```python
from build123d import *

# Parameters (mm, degrees)
BOSS_EXTRU_2_DEPTH        = 6.35
ESQUISSE29_R              = 5
BOSS_EXTRU_3_DEPTH        = 6.35
SYM_TRIE2_COPY_1_SKETCH_R = 5
SYM_TRIE2_COPY_1_DEPTH    = 6.35
ESQUISSE30_R              = 1.5
ENL_V_MAT_EXTRU_1_DEPTH   = 41.953581056


with BuildPart() as part:
    # Esquisse28 → Boss.-Extru.2 (new body)
    with BuildSketch(Plane.XY):
        Polygon((-18.97, -25.475382387), (-25.475382387, -18.97), (-25.475382387, 18.97), (-18.97, 25.475382387), (18.97, 25.475382387), (25.475382387, 18.97), (25.475382387, -18.97), (18.97, -25.475382387), align=None)
        Polygon((-16.97, -20.645541049), (-20.645541049, -16.97), (-20.645541049, 16.97), (-16.97, 20.645541049), (16.97, 20.645541049), (20.645541049, 16.97), (20.645541049, -16.97), (16.97, -20.645541049), align=None, mode=Mode.SUBTRACT)
    extrude(amount=BOSS_EXTRU_2_DEPTH)

    # Esquisse29 → Boss.-Extru.3 (add)
    with BuildSketch(Plane.XY):
        with Locations((23.60833184, 23.60833184)):
            Circle(ESQUISSE29_R)
    boss_extru_3 = extrude(amount=BOSS_EXTRU_3_DEPTH)

    # Symétrie1: Boss.-Extru.3 across plane
    add(boss_extru_3.mirror(Plane(origin=(0, 0, 0), x_dir=(0, 0, 1), z_dir=(1, 0, 0))))

    # Symétrie2: Boss.-Extru.3 across plane
    add(boss_extru_3.mirror(Plane.ZX))

    # Symétrie2 copy 1 sketch → Symétrie2 copy 1 (add)
    with BuildSketch(Plane(origin=(0, 0, 0), x_dir=(-1, 0, 0), z_dir=(0, 0, 1))):
        with Locations((23.60833184, 23.60833184)):
            Circle(SYM_TRIE2_COPY_1_SKETCH_R)
    extrude(amount=SYM_TRIE2_COPY_1_DEPTH)

    # Esquisse30 → Enlèv. mat.-Extru.1 (cut, through all)
    with BuildSketch(Plane.XY.offset(6.35)):
        with Locations((-23.60833184, 23.60833184)):
            Circle(ESQUISSE30_R)
        with Locations((23.60833184, 23.60833184)):
            Circle(ESQUISSE30_R)
        with Locations((23.60833184, -23.60833184)):
            Circle(ESQUISSE30_R)
        with Locations((-23.60833184, -23.60833184)):
            Circle(ESQUISSE30_R)
    extrude(amount=-ENL_V_MAT_EXTRU_1_DEPTH, mode=Mode.SUBTRACT)


solid = part.part
```
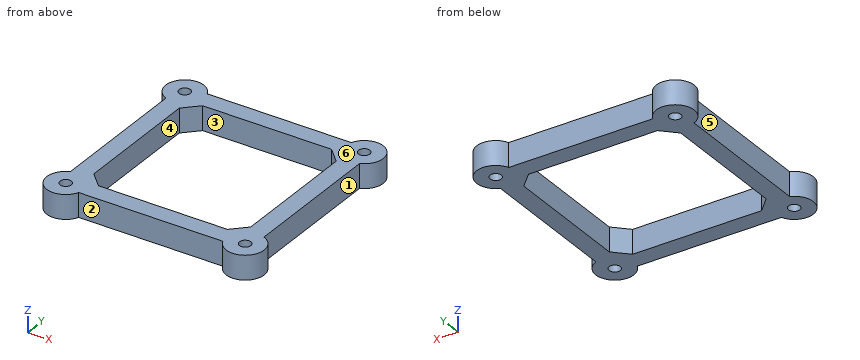
Model file for the job. Use its own axes, mm. Face numbers are marked on the shaded views. A direction names the side the tool comes from. Give positions to 0.01 mm unless a question says otherwise; leave off trailing zeros. Order: outer loops, then holes, each group sorted by start corner. A loop starts at its lowest first (then second) coordinate and runs counter-clockwise, first axis right, second up.
1) Wall check: probe 1 along X at (y, z) = (23.5, 4.75); probe 2 along X at (y, z) = (-15, 2.5). Give the ranges that are in metal, low to high.
2) Saw through at A-A, the plane y = 11. Write the cut outline in (x, z).
3) Pin check, flat tips, straight feed: pin 1 (3 mm diameter, centred on y = -8.5, z = 3.5, fed in from -X); pin 2 (1.8 mm diameter, centred on x = 23.61, y = 23.61, fed in from +Z); pin 3 (2 mm diameter, centred on x = -17.5, z = 2.5, fed in from +Y); pin 4 (5 mm diameter, centred on x = -23.61, y = 23.61, fed in from +Z). Stop position of each tip, or through.
4) Mould opens along X. For the marked faces 4, 5 and 6 say: +X half, -X half, draft (parallel to the pull), parting line (faces both ways), or undercut.
5) Saw through at C-C, the plane z = 2.75. Write the cut outline in (x, y), then the cut area to 3 significant figures.
6) 3-axis set-ups, long thin cutter, end or side, ignore diameter. For the marked faces 1, 2 and 3: which of +Z, -Z, +X, -X, +Y, -Y reach the whole face in a straight line?
Computed:
1. probe 1: x = -28.61 to -25.1, -22.11 to 22.11, 25.1 to 28.61
1. probe 2: x = -25.48 to -20.65, 20.65 to 25.48
2. outline: (-25.48, 0) - (-20.65, 0) - (-20.65, 6.35) - (-25.48, 6.35) - close; (20.65, 0) - (25.48, 0) - (25.48, 6.35) - (20.65, 6.35) - close
3. pin 1: stops at x = -25.48
3. pin 2: passes through
3. pin 3: stops at y = 25.48
3. pin 4: stops at z = 6.35
4. face 4: undercut
4. face 5: -X half
4. face 6: draft
5. outline: (-25.48, -18.97) arc R5 ccw (long way) to (-18.97, -25.48) - (18.97, -25.48) arc R5 ccw (long way) to (25.48, -18.97) - (25.48, 18.97) arc R5 ccw (long way) to (18.97, 25.48) - (-18.97, 25.48) arc R5 ccw (long way) to (-25.48, 18.97) - close; hole circle Ø3 at (-23.61, -23.61); hole circle Ø3 at (-23.61, 23.61); hole (-20.65, -16.97) - (-16.97, -20.65) - (16.97, -20.65) - (20.65, -16.97) - (20.65, 16.97) - (16.97, 20.65) - (-16.97, 20.65) - (-20.65, 16.97) - close; hole circle Ø3 at (23.61, -23.61); hole circle Ø3 at (23.61, 23.61)
5. area: 1,040 mm2
6. face 1: +Z, -Z, +X
6. face 2: +Z, -Z, -Y
6. face 3: +Z, -Z
